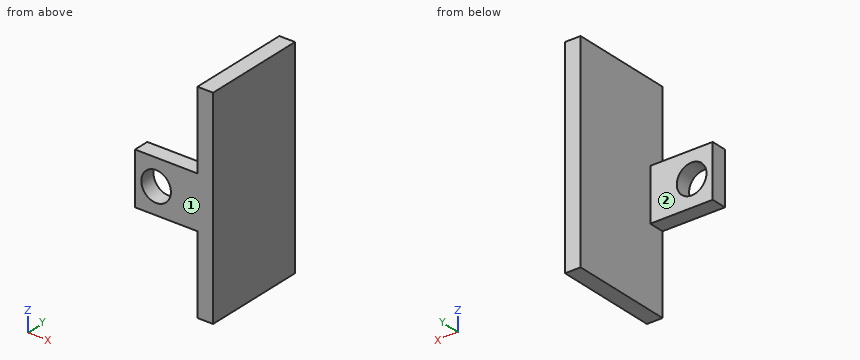
Autodesk Inventor part; units mm, degrees
ref_plane "YZ Plane" through (0, 0, 0) normal (1, 0, 0) x (0, 1, 0)
ref_plane "XZ Plane" through (0, 0, 0) normal (0, 1, 0) x (-1, 0, 0)
ref_plane "XY Plane" through (0, 0, 0) normal (0, 0, 1) x (1, 0, 0)
sketch "Sketch1" plane through (0, 0, 0) normal (0, 1, 0) x (-1, 0, 0)
  line L0 (4.0517, 5) -> (-7.9483, 5)
  line L1 (-7.9483, 5) -> (-7.9483, -5)
  line L2 (-7.9483, -5) -> (4.0517, -5)
  line L3 (4.0517, -5) -> (4.0517, 5)
  circle A0 centre (0, 0) radius 2.85
  dimension "d0" = 5.7
  dimension "d1" = 10
  dimension "d2" = 5
  dimension "d3" = 12
extrude "Extrusion1" add sketch "Sketch1" along normal blind 3
sketch "Sketch2" plane through (7.9483, 0, 5) normal (1, 0, 0) x (0, 0, -1)
  line L0 (-15, 0) -> (25, 0)
  line L1 (25, 0) -> (25, 20)
  line L2 (25, 20) -> (-15, 20)
  line L3 (-15, 20) -> (-15, 0)
  line L4 (0, 0) -> (0, 3)
  line L5 (10, 0) -> (0, 0)
  point P0 (5, 0)
  dimension "d6" = 40
  dimension "d7" = 20
  dimension "d8" = 15
extrude "Extrusion2" add sketch "Sketch2" along normal blind 3
Build history of the part. All positions in model axes, mm. Face numbers are marked on the shaded views. A direction names the side the tool comes from. Coordinates: 2 decimals unless noted, no trailing zeros. Order: outer loops, then holes, each group sorted by start corner. A loop starts at its lowest first (then second) coordinate and runs counter-clockwise, first axis right, second up.
Item 1: Drop flat-ended pins along their axis: pin 1 Ø10 at (y, z) = (5, 0.5) entering from -X; pin 2 Ø2 at (y, z) = (15.5, 11.5) entering from -X; pin 3 Ø1.5 at (x, y) = (0, 1.5) entering from -Z; pin 4 Ø0.9 at (x, y) = (1, 1) entering from +Z. Give the stop position or say it passes through.
Filled in:
pin 1: stops at x = -4.05
pin 2: stops at x = 7.95
pin 3: stops at z = -5
pin 4: stops at z = 5
Item 2: Saw through at C-C on z = -4. List the corners of the cut face in (x, y), then the cut area to 3 significant figures.
Filled in:
outline: (-4.05, 0) - (10.95, 0) - (10.95, 20) - (7.95, 20) - (7.95, 3) - (-4.05, 3) - close
area: 96.0 mm2
Item 3: Tool access for the marked faces 1 and 2: list every direction of +Z, -Z, +X, -X, +Y, -Y with a clear straight run to the whole face (end or side of a thin tool).
Filled in:
face 1: +Z, -Z, +X, -X, -Y
face 2: +Z, -Z, -X, +Y
Item 4: Saw through at A-A on z = 0. List the corners of the cut face in (x, y), then the cut area to 3 significant figures.
Filled in:
outline: (-4.05, 0) - (-2.85, 0) - (-2.85, 3) - (-4.05, 3) - close; (2.85, 0) - (10.95, 0) - (10.95, 20) - (7.95, 20) - (7.95, 3) - (2.85, 3) - close
area: 78.9 mm2
Item 5: Saw through at D-D on y = 18.25. List the corners of the cut face in (x, z).
Filled in:
outline: (7.95, -20) - (10.95, -20) - (10.95, 20) - (7.95, 20) - close
Item 6: Saw through at B-B on x = 0. List the corners of the cut face in (y, z).
Filled in:
outline: (0, -5) - (3, -5) - (3, -2.85) - (0, -2.85) - close; (0, 2.85) - (3, 2.85) - (3, 5) - (0, 5) - close
Item 7: Drill centre lines: L1, parallel to X at y = 13, z = -10; L2, parallel to Z at x = 0, y = 1.9; L3, parallel to Y at x = 5.5, z = 4. Where is each one in solid material? Low to high.
Filled in:
L1: x = 7.95 to 10.95
L2: z = -5 to -2.85, 2.85 to 5
L3: y = 0 to 3
